Job drawing, mm, ordinate dimensions from the low corner. One solid piece. A direction names the side the tool comes from. Give positions to 0.01 mm unless a question says otherwise; leave off trailing zeros. Write each loop counter-clockwise with the first axis right and the second up, starting at its lowest first coordinate (ties: lowest second). Pieces come first, ordered by that corner, then holes. Notation, with made-up numbers: (48, 23.5) - (59, 23.5) arc R22 ccw to (59, 32.5) - close; hole circle Ø10 at (82.25, 57.5). An arc over 180 degrees is marked (long way). Put each result on its own line as item: value. Start each with the question number.
1. Wall check: line 1 (X direction, y = 29, z = 27) (1 decimal); line 2 (Y direction, x = 30, z = 14); line 3 (X direction, y = 5.5, z = 3.5) (1 decimal). Give the ranges that are in metal, low to high.
2. Tool access for the marked faces 4, 5 and 6: list every direction of +Z, -Z, +X, -X, +Y, -Y with a clear straight run to the whole face (end or side of a thin tool).
3. Cut at B-B on z = 25.4. List the corners of the cut face in (x, y) (1 decimal), and give its area (3 significant figures).
4. Cut at D-D on z = 44.5. List the corners of the cut face in (x, y) (1 decimal), and give its area (3 significant figures).
5. Cut at A-A on y = 11. List the corners of the cut face in (x, z) (1 decimal).
6. Cut at C-C on x = 60.5. List the corners of the cut face in (y, z), and give its area (3 significant figures).
7. Mould opens along X. For the marked faces 1, 2 and 3 say: +X half, -X half, draft (parallel to the pull), parting line (faces both ways), or undercut.
8. Drop flat-ended pins along their axis: pin 1 (1.5 mm diameter, centred on x = 46.5, z = 10, fed in from +Y); pin 2 (4 mm diameter, centred on y = 13, z = 12, fed in from +X); pin 3 (6 mm diameter, centred on x = 47.5, z = 18.5, fed in from +Y); pin 4 (8.5 mm diameter, centred on x = 15, y = 19.5, fed in from +Z). Give the stop position or say it passes through.
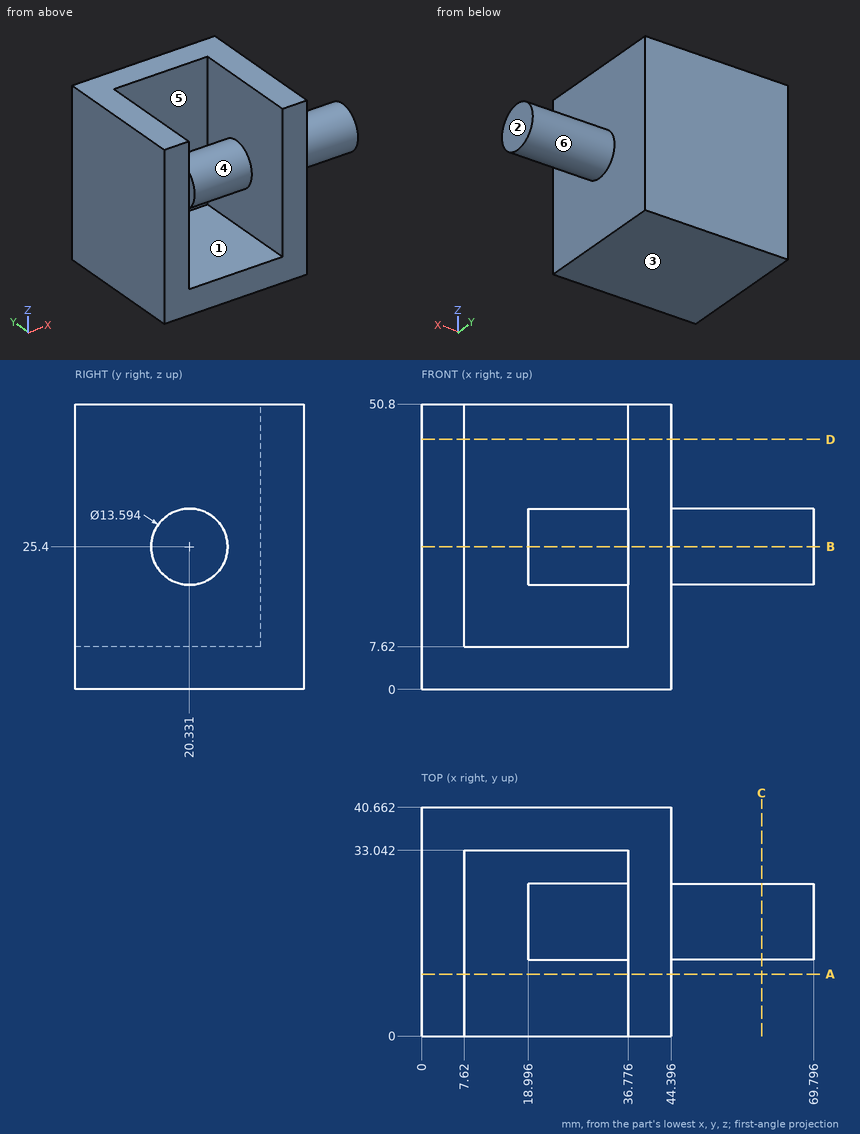
Report:
1. line 1: x = 0 to 7.6, 36.8 to 44.4
1. line 2: y = 33.04 to 40.66
1. line 3: x = 0 to 44.4
2. face 4: none
2. face 5: +Z
2. face 6: +X
3. outline: (0, 0) - (7.6, 0) - (7.6, 33) - (36.8, 33) - (36.8, 27.1) - (19, 27.1) - (19, 13.5) - (36.8, 13.5) - (36.8, 0) - (44.4, 0) - (44.4, 13.5) - (69.8, 13.5) - (69.8, 27.1) - (44.4, 27.1) - (44.4, 40.7) - (0, 40.7) - close
3. area: 1,430 mm²
4. outline: (0, 0) - (7.6, 0) - (7.6, 33) - (36.8, 33) - (36.8, 0) - (44.4, 0) - (44.4, 40.7) - (0, 40.7) - close
4. area: 842 mm²
5. outline: (0, 0) - (44.4, 0) - (44.4, 50.8) - (36.8, 50.8) - (36.8, 7.6) - (7.6, 7.6) - (7.6, 50.8) - (0, 50.8) - close
6. outline: circle Ø13.59 at (20.33, 25.4)
6. area: 145 mm²
7. face 1: undercut
7. face 2: +X half
7. face 3: draft
8. pin 1: passes through
8. pin 2: stops at x = 44.4
8. pin 3: stops at y = 25.9
8. pin 4: stops at z = 32.2
